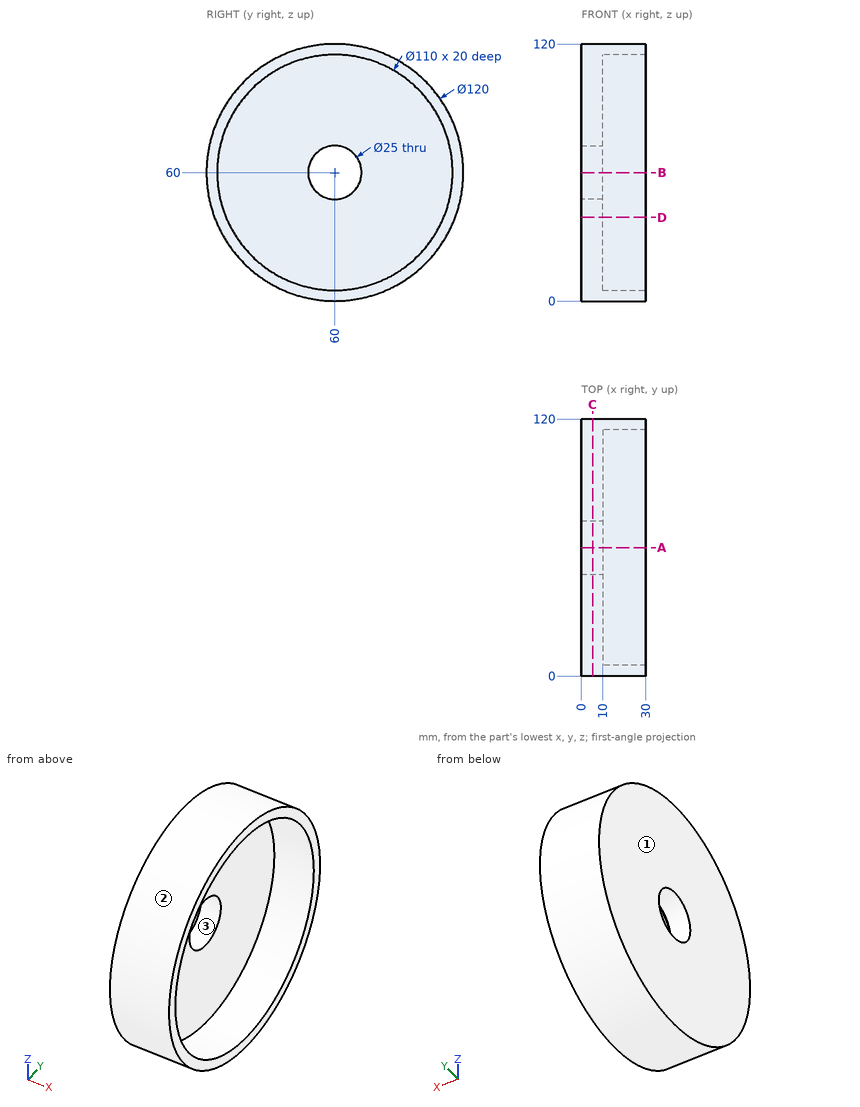
The drawing under review shows one solid part. Ordinate dimensions are in mm from its lowest x, y, z. Round coordinates to 2 decimals unless told otherwise and drop trailing zeros. Write each loop counter-clockwise with the first axis right and the second up, starting at its lowest first coordinate (ties: lowest second). Pieces come first, ordered by that corner, then holes. Notation, with made-up numbers: (-24, 5.25) -> (19, 5.25) arc R32 ccw to (19, 32.25) -> close; hole circle Ø4 at (-9.75, -37.75). An arc over 180 degrees is marked (long way). One line per question, with ' | ' between items. Start each with the question number.
(1) Insertion check: P1, Ø6, axis at x = 26.5, y = 99.5, coming from the -Z side; P2, Ø2, axis at x = 4.5, y = 99, coming from the -Z side; P3, Ø6, axis at x = 6, z = 91.5, coming from the +Y side. Each pin has a flat end and moves straight along its axis. Give the tip position at first contact, or say it passes through.
(2) Add section A-A, the plane y = 60. Write out the cut boundary in (x, z), plus the area to 3 significant figures.
(3) Add section C-C, the plane x = 5.25. Write out the cut boundary in (y, z).
(4) For line 1 along Y through (x, z) = (15, 60); line 2 along Y through (x, z) = (5, 60); line 3 along Z through (x, y) = (22.25, 109), list the stretches that pass through material, from the lowest coordinate up. Write a range as from..to.
(5) Add section D-D, the plane z = 39. Write out the cut boundary in (x, y).
(6) Mouldability with a two-part tool opening along Y and no side actions: class the marked faces 1, 2 and 3 as released by +Y, released by -Y, zero draft, split by the parting line, or undercut.
Answer list:
1) P1: z = 12.38 | P2: z = 13.57 | P3: y = 112.8
2) outline: (0, 0) -> (30, 0) -> (30, 5) -> (10, 5) -> (10, 47.5) -> (0, 47.5) -> close; (0, 72.5) -> (10, 72.5) -> (10, 115) -> (30, 115) -> (30, 120) -> (0, 120) -> close | area: 1,150 mm²
3) outline: circle Ø120 at (60, 60); hole circle Ø25 at (60, 60)
4) line 1: 0..5, 115..120 | line 2: 0..47.5, 72.5..120 | line 3: 25.37..35.02, 84.98..94.63
5) outline: (0, 3.8) -> (30, 3.8) -> (30, 9.17) -> (10, 9.17) -> (10, 110.83) -> (30, 110.83) -> (30, 116.2) -> (0, 116.2) -> close
6) face 1: zero draft | face 2: split by the parting line | face 3: undercut
